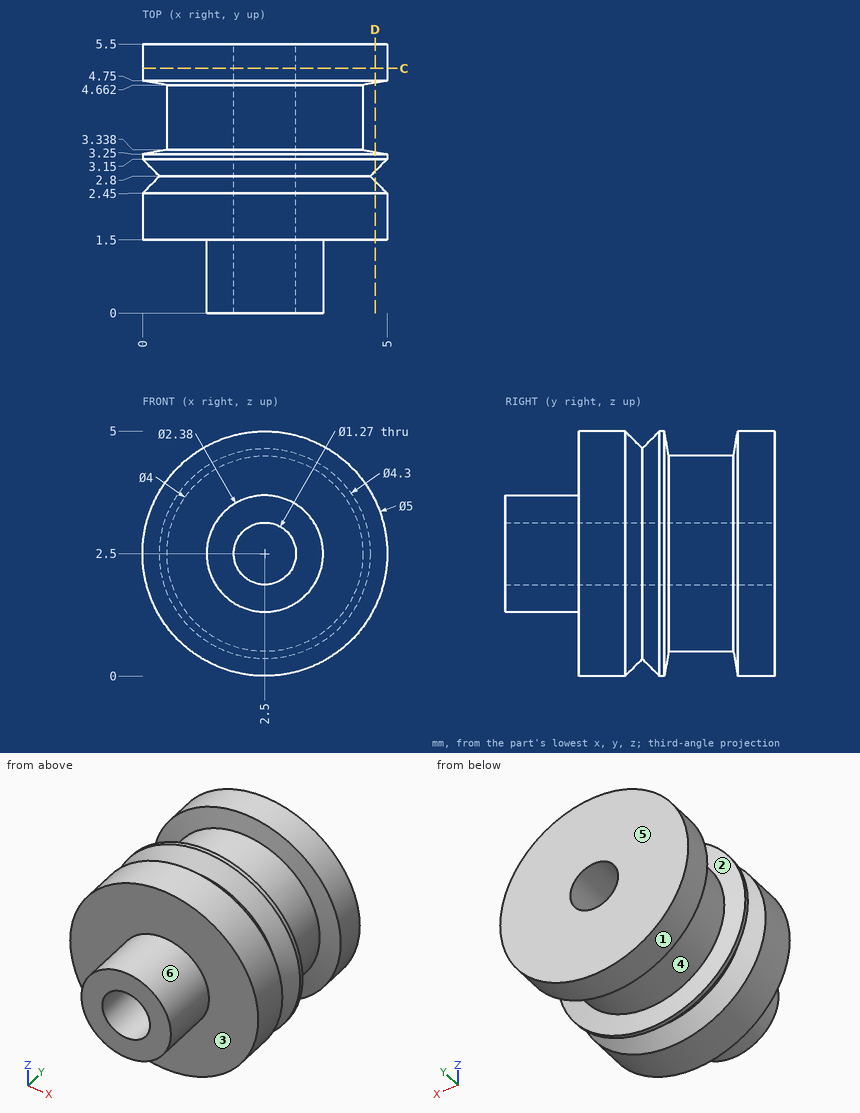
Answer from the drawing. Dimensions are ordinates in mm from the lowest x, y and z of the part. A direction names the side the tool comes from. Coordinates: 2 decimals unless noted, no trailing zeros. Order: outer loops, then holes, each group sorted by start corner. A loop starts at its lowest first (then second) coordinate and runs counter-clockwise, first axis right, second up. Notation, with made-up numbers: (-32.75, 8.25) - (-16.75, 8.25) arc R18 cw to (-16.75, 28.25) - close; hole circle Ø10 at (49.5, 29.25). An arc over 180 degrees is marked (long way). Use one line per item in the form item = value.
(1) Section C-C, the plane y = 5 is taken. Give the vertices of the cut face in (x, z) (3 decimals).
Computed values:
outline = circle Ø5 at (2.5, 2.5); hole circle Ø1.27 at (2.5, 2.5)
(2) For a pull along Y with two mould halves and no side action, classify the marked faces 4, 5 and 6 as pulls with the +Y half, pulls with the -Y half, needs draft (parallel to the pull), parting line crosses it, or undercut.
Computed values:
face_4 = undercut
face_5 = pulls with the +Y half
face_6 = needs draft
(3) Which of the six approach directions +Z, -Z, +X, -X, +Y, -Y give full straight-line access (tool end or side, diameter ignored) to the marked faces 1, 2 and 3?
Computed values:
face_1 = +Y, -Y
face_2 = none
face_3 = -Y
(4) Straight lines are drawn through the part: L1, parallel to X at y = 3.2, z = 2.5 (3 decimals); L2, parallel to Z at x = 2.5, y = 1.3 (3 decimals). For each, find the intervals that lie inside material, in ascending order.
Computed values:
L1 = 0 to 1.865, 3.135 to 5
L2 = 1.31 to 1.865, 3.135 to 3.69
(5) Section D-D, the plane x = 4.75 is taken. Give the number of separate pieces and of enclosed holes in the cut face.
Computed values:
separate_pieces = 3
enclosed_holes = 0
(6) Given pin 1 Ø2 at (x, z) = (1.5, 1.5) entering from -Y, flat-ended and moving along its own axis, determine where the tip first touches the part or whether it passes through.
Computed values:
pin_1 = 0
